from build123d import *

# Parameters (mm, degrees)
F1_DEPTH = 34.544
F3_D     = 4.1
F3_DEPTH = 12.7
F3_TIP   = 1.231764269


with BuildPart() as f1:
    # F0 (on Top) → F1 (new body, symmetric)
    with BuildSketch(Plane.XY):
        Polygon((-13.8865606859, 60.4830309749), (-42.757101357, 23.3497414738), (-11.2690485742, -15.0952798912), (-5.2401868215, -50.4424741696), (38.2038913667, -43.0325977504), (25.8125865485, 29.6175768167), align=None)
    extrude(amount=F1_DEPTH, both=True)

    # F3
    with Locations(Plane.XY.offset(34.544)):
        with Locations((-15.0234112516, 48.1616705656), (-24.3386197835, 30.192643404), (21.6382276267, -23.181784898)):
            Hole(F3_D / 2, depth=F3_DEPTH)
            with Locations((0, 0, -(F3_DEPTH + F3_TIP / 2))):  # 118° drill point
                Cone(0, F3_D / 2, F3_TIP, mode=Mode.SUBTRACT)


solid = f1.part
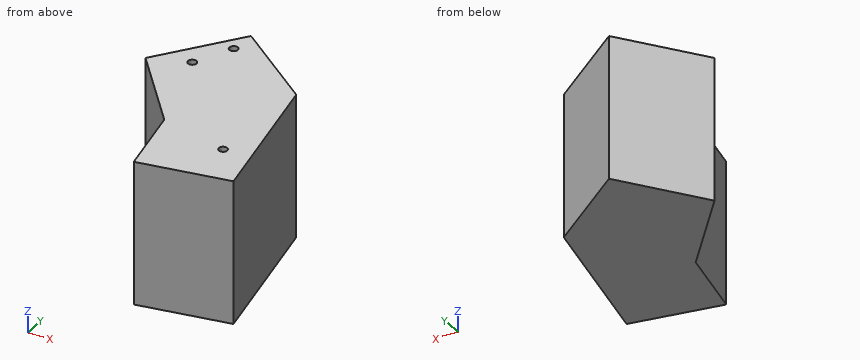
Part model, mm, in its own coordinate system. Give positions to 0.01 mm unless a question says otherwise; leave off trailing zeros. Order: outer loops, then holes, each group sorted by start corner. A loop starts at its lowest first (then second) coordinate and runs counter-clockwise, first axis right, second up. Notation, with made-up numbers: (64, 12) -> (98, 12) arc R24 cw to (98, 36) -> close; hole circle Ø4 at (-35, 35.25). An arc over 180 degrees is marked (long way). Use one line per item in the form item = value.
(1) Flat gauge pins, fed straight in: P1, Ø4, axis at y = 21, z = 10, coming from the +X side; P2, Ø6, axis at y = -10, z = 26.5, coming from the +X side; P3, Ø5, axis at x = -2, z = 11, coming from the -Y side. Where does each tip first touch, or does it go through?
Solution:
P1 = 27.62
P2 = 33.08
P3 = -50.32
(2) Saw through at A-A (z = -5.5). Write the cut outline in (x, y).
Solution:
outline = (-42.76, 23.35) -> (-11.27, -15.1) -> (-5.24, -50.44) -> (38.2, -43.03) -> (25.81, 29.62) -> (-13.89, 60.48) -> close
(3) Saw through at D-D (x = -20.5). Write the cut outline in (y, z), then the cut area to 3 significant figures.
Solution:
outline = (-3.82, -34.54) -> (51.98, -34.54) -> (51.98, 34.54) -> (-3.82, 34.54) -> close
area = 3,860 mm²
(4) Saw through at C-C (y = 54). Write the cut outline in (x, z), then the cut area to 3 significant figures.
Solution:
outline = (-18.93, -34.54) -> (-5.55, -34.54) -> (-5.55, 34.54) -> (-18.93, 34.54) -> close
area = 924 mm²
(5) Saw through at B-B (z = 28). Write the cut outline in (x, y), then the cut area to 3 significant figures.
Solution:
outline = (-42.76, 23.35) -> (-11.27, -15.1) -> (-5.24, -50.44) -> (38.2, -43.03) -> (25.81, 29.62) -> (-13.89, 60.48) -> close; hole circle Ø4.1 at (-24.34, 30.19); hole circle Ø4.1 at (-15.02, 48.16); hole circle Ø4.1 at (21.64, -23.18)
area = 4,970 mm²
(6) Drill centre lines: line 1 (Y direction, x = 1, z = -6); line 2 (Y direction, x = -33.5, z = 27.5); line 3 (X direction, y = 52, z = -20.5). Where is each one in solid material? Low to high. Write a range as from..to.
Solution:
line_1 = -49.38..48.91
line_2 = 12.05..35.26
line_3 = -20.48..-2.98
